```python
from build123d import *
from OCP.BRepFilletAPI import BRepFilletAPI_MakeChamfer

# Parameters (mm, degrees)
SKETCH1_W           = 110
SKETCH1_H           = 69
BOSS_EXTRUDE1_DEPTH = 3
CHAMFER1_SIZE       = 2
CHAMFER1_SIZE2      = 3.5
FILLET1_R           = 1
SKETCH2_R           = 1.5
BOSS_EXTRUDE2_DEPTH = 0.5


with BuildPart() as part:
    # Sketch1 → Boss-Extrude1 (new body)
    with BuildSketch(Plane(origin=(0, 0, 0), x_dir=(1, 0, 0), z_dir=(0, 1, 0))):
        Rectangle(SKETCH1_W, SKETCH1_H)
    extrude(amount=BOSS_EXTRUDE1_DEPTH)

    # Chamfer1: one chamfer whose edges measure the first distance from different faces: ONE call of the kernel's chamfer builder (chamfer() names one face for all edges)
    chamfer1_edges_1 = [part.edges().sort_by_distance(p)[0] for p in [
        (-55, 3, 0),
    ]]
    chamfer1_side_1 = [part.faces().sort_by_distance(p)[0] for p in [
        (-55, 1.5, 0),
    ]]
    chamfer1_edges_2 = [part.edges().sort_by_distance(p)[0] for p in [
        (0, 3, 34.5),
    ]]
    chamfer1_side_2 = [part.faces().sort_by_distance(p)[0] for p in [
        (0, 1.5, 34.5),
    ]]
    chamfer1_edges_3 = [part.edges().sort_by_distance(p)[0] for p in [
        (55, 3, 0),
    ]]
    chamfer1_side_3 = [part.faces().sort_by_distance(p)[0] for p in [
        (55, 1.5, 0),
    ]]
    chamfer1_edges_4 = [part.edges().sort_by_distance(p)[0] for p in [
        (0, 3, -34.5),
    ]]
    chamfer1_side_4 = [part.faces().sort_by_distance(p)[0] for p in [
        (0, 1.5, -34.5),
    ]]
    chamfer1 = BRepFilletAPI_MakeChamfer(part.part.solid().wrapped)
    for e in chamfer1_edges_1:
        chamfer1.Add(CHAMFER1_SIZE, CHAMFER1_SIZE2, e.wrapped, chamfer1_side_1[0].wrapped)  # the first distance lies on this face
    for e in chamfer1_edges_2:
        chamfer1.Add(CHAMFER1_SIZE, CHAMFER1_SIZE2, e.wrapped, chamfer1_side_2[0].wrapped)  # the first distance lies on this face
    for e in chamfer1_edges_3:
        chamfer1.Add(CHAMFER1_SIZE, CHAMFER1_SIZE2, e.wrapped, chamfer1_side_3[0].wrapped)  # the first distance lies on this face
    for e in chamfer1_edges_4:
        chamfer1.Add(CHAMFER1_SIZE, CHAMFER1_SIZE2, e.wrapped, chamfer1_side_4[0].wrapped)  # the first distance lies on this face
    add(Compound.cast(chamfer1.Shape()), mode=Mode.REPLACE)

    # Fillet1
    fillet1_edges = [part.edges().sort_by_distance(p)[0] for p in [
        (51.5, 3, 0),
        (0, 3, -31),
        (-51.5, 3, 0),
        (0, 3, 31),
    ]]
    fillet(fillet1_edges, radius=FILLET1_R)

    # Sketch2 → Boss-Extrude2 (add)
    with BuildSketch(Plane.XZ):
        with Locations(Location((44, 3.5, 0), (0, 0, 90))):
            Circle(SKETCH2_R)
        with Locations(Location((44, -3.5, 0), (0, 0, 90))):
            Circle(SKETCH2_R)
    extrude(amount=BOSS_EXTRUDE2_DEPTH)


solid = part.part
```
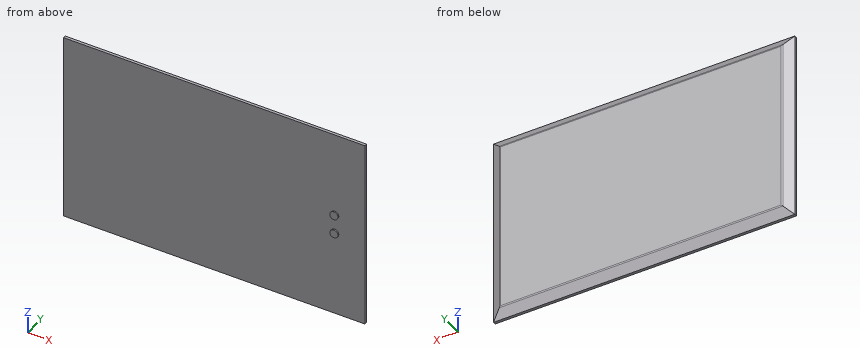
The listing builds one solid part. Answer for the finished solid, in the listing's coordinates (mm). Coordinates: 2 decimals unless noted, no trailing zeros. Loops run counter-clockwise (first coordinate to the right, second up) from the corner with the lowest first, then second, coordinate; pieces in that order, holes last. Notation, with made-up numbers: M 5,-37 L 25,-37 A17 cw 25,-22 Z; hole C -31,17 d1. An arc over 180 degrees is marked long. Answer as a JSON object with one key per item and string values. Group by question number.
Item 1: Section B-B (x = -17) is taken. Write down the section's boundary in (y, z).
Item 2: Section A-A (z = -25.5) is taken. Write down the section's boundary in (x, y), and give its area (3 significant figures).
Item 3: Section C-C (y = 1.8) is taken. Write down the section's boundary in (x, z), and give its area (3 significant figures).
Item 4: Section D-D (z = 3.5) is taken. Write down the section's boundary in (x, y).
Item 5: Consider L1, parallel to Y at x = 42, z = 4.5; L2, parallel to X at y = 1.4, z = -17; L3, parallel to X at y = 2.5, z = 6.5 (3 decimals). Determine where each line is inside the solid, lowest interval first.
Item 6: This flat-tipped pin is pushed along its axis until it touches: P1, Ø8, axis at x = 1.5, z = -2, coming from the -Y side. Where does it stop, or does it pass through?
Solved:
{
 "1": {"outline": "M 0,-34.5 L 1,-34.5 L 2.87,-31.23 A1 ccw 3,-30.73 L 3,30.73 A1 ccw 2.87,31.23 L 1,34.5 L 0,34.5 Z"},
 "2": {"outline": "M -55,0 L 55,0 L 55,1 L 51.73,2.87 A1 ccw 51.23,3 L -51.23,3 A1 ccw -51.73,2.87 L -55,1 Z", "area": "323 mm2"},
 "3": {"outline": "M -53.6,-33.1 L 53.6,-33.1 L 53.6,33.1 L -53.6,33.1 Z", "area": "7,100 mm2"},
 "4": {"outline": "M -55,0 L 42.5,0 L 42.5,-0.5 L 45.5,-0.5 L 45.5,0 L 55,0 L 55,1 L 51.73,2.87 A1 ccw 51.23,3 L -51.23,3 A1 ccw -51.73,2.87 L -55,1 Z"},
 "5": {"L1": "y = 0 to 3", "L2": "x = -54.3 to 54.3", "L3": "x = -52.375 to 52.375"},
 "6": {"P1": "stops at y = 0"}
}
